Read the model definition and answer for the solid it produces. Units are mm, in the model's axes. Give positions to 0.01 mm unless a question says otherwise; leave off trailing zeros. Order: outer loops, then holes, each group sorted by start corner. A loop starts at its lowest first (then second) coordinate and runs counter-clockwise, first axis right, second up. Notation, with made-up numbers: M -12,46 L 30,46 A19 ccw 30,60 Z; hole C 80,21 d11. An arc over 180 degrees is marked long. One line per item, written item: value.
Solid Edge part; units mm, degrees
sketch "Sketch1" plane through (0, 0, 0) normal (0, 0, 1) x (1, 0, 0)
  line L0 (-3.675, 6.3653) -> (3.675, 6.3653)
  line L1 (3.675, 6.3653) -> (7.35, 0)
  line L2 (7.35, 0) -> (3.675, -6.3653)
  line L3 (3.675, -6.3653) -> (-3.675, -6.3653)
  line L4 (-3.675, -6.3653) -> (-7.35, 0)
  line L5 (-7.35, 0) -> (-3.675, 6.3653)
extrude "Protrusion1" add sketch "Sketch1" along normal mid plane 6.4
sketch "Sketch2" plane through (0, -5.5125, 6.3) normal (-1, 0, 0) x (0, 1, 0)
  line L0 (-2.267, 7.8858) -> (0.5614, 10.7142)
  line L1 (-2.267, 7.8858) -> (-2.267, 4.7142)
  line L2 (-2.267, 4.7142) -> (0.5614, 1.8858)
revolve "RevolvedCutout1" cut sketch "Sketch2" angle 360 about axis through (0, 0, 0.5943) along (0, 0, -1) material side at (0, -6.4007, -3.0354)
hole "Hole_1" at (0, 0, 3.2) direction (0, 0, -1) diameter 6.647 end up to next
properties material "Stainless steel"
1) Find section A-A, the plane x = 0. Write down the section's boundary in (y, z).
Reported:
outline: M -6.37,-3 L -6.17,-3.2 L -3.32,-3.2 L -3.32,3.2 L -6.17,3.2 L -6.37,3 Z; M 3.32,-3.2 L 6.17,-3.2 L 6.37,-3 L 6.37,3 L 6.17,3.2 L 3.32,3.2 Z
2) Consider probe 1 along Y at (x, z) = (0, -0.75); probe 2 along Y at (x, z) = (-3, -2.25); probe 3 along X at (y, z) = (-2.25, 0). Determine where each line is inside the solid, lowest interval first.
Reported:
probe 1: y = -6.37 to -3.32, 3.32 to 6.37
probe 2: y = -6.37 to -1.43, 1.43 to 6.37
probe 3: x = -6.05 to -2.45, 2.45 to 6.05
3) Find section C-C, the plane z = 2.5. Write down the section's boundary in (x, y), plus the area to 3 significant figures.
Reported:
outline: M -6.8,-0.96 L -4.23,-5.41 A6.87 ccw -2.57,-6.37 L 2.57,-6.37 A6.87 ccw 4.23,-5.41 L 6.8,-0.96 A6.87 ccw 6.8,0.96 L 4.23,5.41 A6.87 ccw 2.57,6.37 L -2.57,6.37 A6.87 ccw -4.23,5.41 L -6.8,0.96 A6.87 ccw Z; hole C 0,0 d6.65
area: 103 mm^2
4) Determine the mould class of faces 1 (the face through (0, 6.365, 0)), 2 (the face through (-1.27, -3.07, 0.04)), 3 (the face through (5.487, 3.227, -0.042)) for opening direction X: +X half, -X half, draft (parallel to the pull), parting line (faces both ways), or undercut.
Reported:
face 1: draft
face 2: undercut
face 3: +X half
5) Each of these flat-tipped pins is pushed along its axis until it touches: pin 1 Ø2 at (y, z) = (-2, -2) entering from -X; pin 2 Ø1.5 at (y, z) = (-4.5, 0.5) entering from -X. Where does it stop, or does it pass through?
Reported:
pin 1: stops at x = -6.77
pin 2: stops at x = -5.18
